Autodesk Inventor part; units mm, degrees
ref_plane "Work Plane2" through (-6.35, 50, -25.4) normal (0.5, 0.866, 0) x (0, 0, 1)
ref_plane "Work Plane3" through (124.1493, 263.3314, 0.1214) normal (0, 1, 0) x (0, 0, -1)
ref_plane "YZ Plane" through (0, 0, 0) normal (1, 0, 0) x (0, 1, 0)
sketch "Sketch1" plane through (0, 0, 0) normal (0, 1, 0) x (-1, 0, 0)
  line L0 (0, 0) -> (6.35, 0)
  line L1 (6.35, 0) -> (6.35, -25.4)
  line L2 (6.35, -25.4) -> (0, -25.4)
  line L3 (0, -25.4) -> (0, 0)
  dimension "d0" = 6.35
  dimension "d1" = 25.4
extrude "Extrusion1" add sketch "Sketch1" along normal blind 50
sketch "Sketch2" plane through (0, 50, 0) normal (0, 1, 0) x (1, 0, 0)
  point P0 (0, 0)
ref_plane "Work Plane2" through (-6.35, 50, -25.4) normal (0.5, 0.866, 0) x (0, 0, 1)
sketch "Sketch3" plane through (-6.35, 50, -25.4) normal (0.5, 0.866, 0) x (0, 0, 1)
  line L0 (25.5214, 0) -> (0.1214, 0)
  line L1 (0.1214, 0) -> (0.1214, 6.35)
  line L2 (0.1214, 6.35) -> (25.5214, 6.35)
  line L3 (25.5214, 6.35) -> (25.5214, 0)
  point P0 (25.4, 30.4993)
  dimension "d5" = 25.4
  dimension "d6" = 6.35
extrude "Extrusion2" add sketch "Sketch3" along normal blind 250
ref_plane "Work Plane3" through (124.1493, 263.3314, 0.1214) normal (0, 1, 0) x (0, 0, -1)
sketch "Sketch4" plane through (124.1493, 263.3314, 0.1214) normal (0, 1, 0) x (0, 0, -1)
  line L0 (25.4, 124.1493) -> (25.4, 0)
  line L1 (25.4, 0) -> (0, 0)
  line L2 (0, 0) -> (0, 6.35)
  line L3 (0, 6.35) -> (25.4, 6.35)
  line L4 (25.4, 6.35) -> (25.4, 0)
  point P0 (0.1214, 124.1493)
  point P1 (25.4, 6.35)
  dimension "d10" = 25.4
  dimension "d11" = 6.35
extrude "Extrusion3" add sketch "Sketch4" along normal blind 50
mirror "Mirror1" about plane through (120.9743, 313.3314, -12.5786) normal (0, 1, 0) of "Extrusion1", "Extrusion2", "Extrusion3"
properties part number "AçoChato"
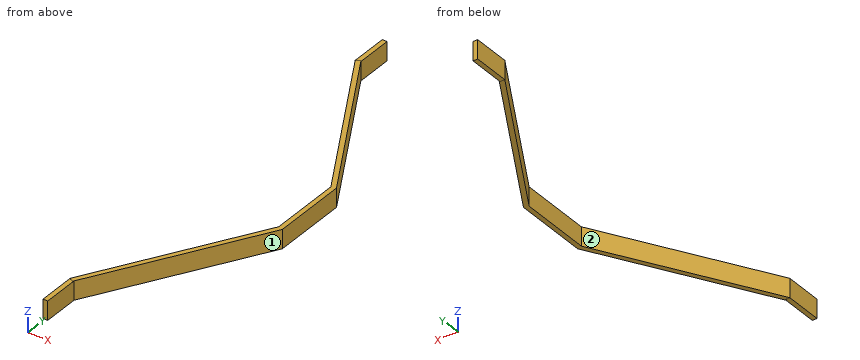
Part model, mm, in its own coordinate system. Face numbers are marked on the shaded views. Give positions to 0.01 mm unless a question says otherwise; leave off trailing zeros. Write each loop counter-clockwise with the first axis right and the second up, starting at its lowest first coordinate (ties: lowest second). Pieces come first, ordered by that corner, then holes.
1) Cut at A-A on x = 92. Write the cut outline in (y, z).
Resolved:
outline: (207.65, -25.28) - (220.35, -25.28) - (220.35, 0.12) - (207.65, 0.12) - close; (406.32, -25.28) - (419.02, -25.28) - (419.02, 0.12) - (406.32, 0.12) - close
2) Cut at C-C on y = 314. Write the cut outline in (x, z).
Resolved:
outline: (117.8, -25.28) - (124.15, -25.28) - (124.15, 0.12) - (117.8, 0.12) - close
3) Pin check, flat tips, straight feed: pin 1 (12.5 mm diameter, centred on y = 25, z = -17, fed in from +X); pin 2 (8 mm diameter, centred on x = 78, z = -20.5, fed in from -Y); pin 3 (3 mm diameter, centred on x = -4, y = 596.5, fed in from +Z). Stop position of each tip, or through.
Resolved:
pin 1: stops at x = 0
pin 2: stops at y = 176.47
pin 3: stops at z = 0
4) Probe L1, parallel to X at y = 298, z = -22.5; L2, parallel to Y at x = 13, z = -11; L3, parallel to Y at x = 114.5, z = -9.75. List the from-to ranges inside material, lowest first.
Resolved:
L1: x = 117.8 to 124.15
L2: y = 70.82 to 83.52, 543.15 to 555.85
L3: y = 246.62 to 259.32, 367.34 to 380.04
5) Two-plate mould, pull along Y, no slides. Class the marked faces 1 and 2: released by +Y, released by -Y, zero draft, split by the parting line, or undercut.
Resolved:
face 1: released by -Y
face 2: undercut
6) Cut at D-D on y = 89. Write the cut outline in (x, z), then the cut area to 3 significant figures.
Resolved:
outline: (16.17, -25.28) - (23.5, -25.28) - (23.5, 0.12) - (16.17, 0.12) - close
area: 186 mm2
